Read the model definition and answer for the solid it produces. Units are mm, in the model's axes. Face numbers are marked on the shaded views. A direction names the side the tool comes from. Coordinates: 2 decimals unless noted, no trailing zeros. Write each loop counter-clockwise with the first axis right and the second up, starting at its lowest first coordinate (ties: lowest second). Pieces come first, ordered by that corner, then holes. Notation, with made-up numbers: (19, 81) -> (72, 81) arc R16 cw to (72, 101) -> close; hole circle Ø6 at (50.5, 28.5). An arc over 180 degrees is marked (long way). Use CSV: the item, a comma, the result in double quotes.
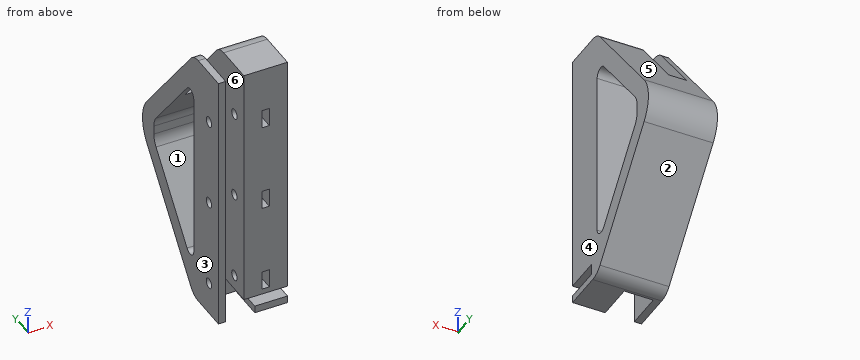
Autodesk Inventor part; units mm, degrees
ref_plane "YZ Plane" through (0, 0, 0) normal (1, 0, 0) x (0, 1, 0)
ref_plane "XZ Plane" through (0, 0, 0) normal (0, 1, 0) x (-1, 0, 0)
ref_plane "XY Plane" through (0, 0, 0) normal (0, 0, 1) x (1, 0, 0)
sketch "Sketch1" plane through (0, 0, 0) normal (0, 1, 0) x (-1, 0, 0)
  line L0 (0, 0) -> (-19, 0)
  line L1 (-19, 0) -> (-19, -73)
  line L2 (-19, -73) -> (0, -73)
  line L3 (0, -73) -> (0, 0)
  dimension "d0" = 19
  dimension "d1" = 73
extrude "Extrusion1" add sketch "Sketch1" along normal blind 13
sketch "Sketch2" plane through (19, 0, 0) normal (1, 0, 0) x (0, 0, -1)
  line L0 (0, 13) -> (0, 43) construction
  line L1 (0, 43) -> (205, 43) construction
  line L2 (0, 13) -> (0, 13.5) construction
  line L3 (0, 0) -> (0, 13) construction
  line L4 (0, 13) -> (0, 13) construction
  line L5 (0, 13) -> (73, 13) construction
  line L6 (0, 13) -> (0, 13) construction
  line L7 (0, 13) -> (73, 13) construction
  line L8 (0, 13) -> (73, 13) construction
  line L9 (36.5, 13) -> (36.5, 43) construction
  line L10 (36.5, 43) -> (0, 13) construction
  line L11 (73, 13) -> (36.5, 43) construction
  line L12 (36.5, 43) -> (30.3197, 37.9203) construction
  line L13 (30.3197, 37.9203) -> (33.4945, 34.0576) construction
  line L14 (33.4945, 34.0576) -> (7.8744, 13) construction
  line L15 (36.5, 43) -> (42.6803, 37.9203) construction
  line L16 (42.6803, 37.9203) -> (39.5055, 34.0576) construction
  line L17 (33.4945, 34.0576) -> (39.5055, 34.0576)
  line L18 (36.5, 43) -> (0, 13)
  line L19 (0, 13) -> (7.8744, 13)
  line L20 (7.8744, 13) -> (33.4945, 34.0576)
  line L21 (73, 13) -> (0, 13) construction
  line L22 (73, 13) -> (0, 13) construction
  line L23 (73, 13) -> (0, 13) construction
  line L24 (36.5, 43) -> (73, 13) construction
  line L25 (39.5055, 34.0576) -> (65.1256, 13) construction
  line L26 (36.5, 43) -> (73, 13)
  line L27 (73, 13) -> (65.1256, 13)
  line L28 (65.1256, 13) -> (39.5055, 34.0576)
  dimension "d4" = 30
  dimension "d5" = 205
  dimension "d6" = 0.5
  dimension "d7" = 0
  dimension "d8" = 0
  dimension "d9" = 73
  dimension "d10" = 0
  dimension "d11" = 8
  dimension "d12" = 5
  dimension "d13" = 8
  dimension "d14" = 5
extrude "Extrusion2" add sketch "Sketch2" against normal up to surface (19 mm away)
fillet "Fillet1" radius 10 1 edges at (9.5, 43, -36.5)
fillet "Fillet4" radius 2 2 edges at (9.5, 13, -7.8744) (9.5, 13, -65.1256)
fillet "Fillet5" radius 5 2 edges at (9.5, 13, -73) (9.5, 13, 0)
sketch "Sketch3" plane through (0, 0, 0) normal (0, -1, 0) x (1, 0, 0)
  line L0 (0, -73) -> (0, 0) construction
  line L1 (0, -73) -> (2, -73) construction
  line L2 (19, -73) -> (0, -73) construction
  line L3 (2, -73) -> (2, 0)
  line L4 (0, 0) -> (19, 0)
  line L5 (2, -73) -> (7, -73) construction
  line L6 (7, -73) -> (7, 0)
  line L7 (7, -73) -> (80, -73) construction
  line L8 (7, -73) -> (2, -73)
  line L9 (7, 0) -> (2, 0)
  dimension "d24" = 2
  dimension "d25" = 5
  dimension "d26" = 90
extrude "Extrusion3" cut sketch "Sketch3" against normal blind 10
sketch "Sketch5" plane through (0, 10, 0) normal (0, -1, 0) x (1, 0, 0)
  line L0 (7, 0) -> (7, -73)
  line L1 (2, -73) -> (2, 0)
  line L2 (7, 0) -> (2, 0)
  line L3 (2, 0) -> (2, -18)
  line L4 (2, -18) -> (7, -18)
  line L5 (7, -18) -> (7, 0)
  point P0 (0, 0)
  dimension "d31" = 18
extrude "Extrusion5" cut sketch "Sketch5" against normal up to next
sketch "Sketch6" plane through (0, 0, -73) normal (-1, 0, 0) x (0, 0, 1)
  circle A0 centre (9.0852, 5) radius 1.4
  circle A1 centre (33.5852, 5) radius 1.4
  circle A2 centre (58.0852, 5) radius 1.4
  point P0 (73, 0)
extrude "Extrusion6" cut sketch "Sketch6" against normal blind 11.995
sketch "Sketch9" plane through (11.995, 5, -14.9148) normal (-1, 0, 0) x (0, 0, 1)
  circle A0 centre (0, 0) radius 3.002 construction
  circle A1 centre (0, 0) radius 1.4 construction
  line L0 (0, 0) -> (0, 3.002) construction
  line L1 (0, 3.002) -> (2.5998, 1.501)
  line L2 (2.5998, 1.501) -> (2.5998, -1.501)
  line L3 (2.5998, -1.501) -> (0, -3.002)
  line L4 (0, -3.002) -> (-2.5998, -1.501)
  line L5 (-2.5998, -1.501) -> (-2.5998, 1.501)
  line L6 (-2.5998, 1.501) -> (0, 3.002)
  line L7 (-58.0852, -5) -> (14.9148, -5)
  line L8 (-2.5998, -1.501) -> (-2.5998, -5)
  line L9 (14.9148, -5) -> (-58.0852, -5)
  line L10 (2.5998, -1.501) -> (2.5998, -5)
  line L11 (2.5998, -1.501) -> (6.0988, -1.501) construction
  line L12 (2.5998, -5) -> (-2.5998, -5)
  dimension "d38" = 6.004
  dimension "d41" = 90
extrude "Extrusion7" cut sketch "Sketch9" against normal blind 2.005
sketch "Sketch10" plane through (14, 5, -14.9148) normal (-1, 0, 0) x (0, 0, 1)
  circle A0 centre (0, 0) radius 1.4
  line L0 (2.5998, -5) -> (-2.5998, -5)
  line L1 (2.5998, 1.501) -> (2.5998, -5)
  line L2 (0, 3.002) -> (2.5998, 1.501)
  line L3 (-2.5998, 1.501) -> (0, 3.002)
  line L4 (-2.5998, -5) -> (-2.5998, 1.501)
  point P0 (14.9148, -5)
extrude "Extrusion8" cut sketch "Sketch10" against normal blind 2 contours A0
ref_plane "Work Plane3" through (0, 5, -14.9148) normal (0, 0, -1) x (1, 0, 0)
ref_plane "Work Plane4" through (0, 5, -39.4148) normal (0, 0, 1) x (1, 0, 0)
ref_plane "Work Plane5" through (0, 5, -63.9148) normal (0, 0, -1) x (1, 0, 0)
ref_plane "Work Plane6" through (0, 5, -27.1648) normal (0, 0, -1) x (1, 0, 0)
ref_plane "Work Plane7" through (0, 5, -51.6648) normal (0, 0, 1) x (1, 0, 0)
mirror "Mirror3" about plane through (0, 5, -27.1648) normal (0, 0, -1) of "Extrusion8", "Extrusion7"
mirror "Mirror4" about plane through (0, 5, -51.6648) normal (0, 0, 1) of "Mirror3"
fillet "Fillet6" radius 5 2 edges at (9.5, 34.0576, -39.5055) (9.5, 34.0576, -33.4945)
sketch "Sketch11" plane through (0, 0, 0) normal (0, -1, 0) x (1, 0, 0)
  line L0 (7, -73) -> (2, -73) construction
  line L1 (7, -73) -> (7, -71) construction
  line L2 (7, -73) -> (9, -73) construction
  line L3 (19, -42.8497) -> (19, -71.1748)
  line L4 (7, -71) -> (19, -71)
  line L5 (19, -71) -> (19, -68)
  line L6 (19, -68) -> (7, -68)
  line L7 (7, -68) -> (7, -71)
  point P0 (0, 0)
  dimension "d48" = 2
  dimension "d49" = 90
  dimension "d50" = 3
extrude "Extrusion9" cut sketch "Sketch11" against normal blind 10
sketch "Sketch12" plane through (19, 10.6374, -73) normal (0, 0, -1) x (-1, 0, 0)
  line L0 (12, -10.6374) -> (0, -10.6374)
  line L1 (0, -0.6374) -> (12, -0.6374)
  line L2 (12, -10.6374) -> (9, -10.6374)
  line L3 (9, -10.6374) -> (9, -0.6374)
  line L4 (9, -0.6374) -> (12, -0.6374)
  line L5 (12, -0.6374) -> (12, -10.6374)
  point P0 (19, -10.6374)
  dimension "d53" = 3
extrude "Extrusion10" cut sketch "Sketch12" against normal up to next
properties part number "bumper_backright"
1. For a pull along X with two mould halves and no side action, classify the marked faces 3, 4, 5 and 6 as pulls with the +X half, pulls with the -X half, needs draft (parallel to the pull), parting line crosses it, or undercut.
Solutions:
face 3,"pulls with the -X half"
face 4,"pulls with the +X half"
face 5,"needs draft"
face 6,"undercut"
2. A cutting plane is placed at C-C (x = 8). Give the vertices of the cut face in (y, z), and give its area (3 significant figures).
Solutions:
outline,"(0, -68) -> (10, -68) -> (10, -73) -> (10.64, -73) arc R5 ccw to (14.5, -71.17) -> (37.78, -42.85) arc R10 ccw to (37.78, -30.15) -> (14.5, -1.83) arc R5 ccw to (10.64, 0) -> (0, 0) -> close; hole circle Ø2.8 at (5, -63.91); hole circle Ø2.8 at (5, -39.41); hole circle Ø2.8 at (5, -14.91); hole (13, -59.54) arc R2 ccw to (16.55, -60.81) -> (32.92, -40.89) arc R5 ccw to (34.06, -37.71) -> (34.06, -35.29) arc R5 ccw to (32.92, -32.11) -> (16.55, -12.19) arc R2 ccw to (13, -13.46) -> close"
area,"1,310 mm^2"
3. A cutting plane is placed at B-B (y = 29.5). Give the vertices of the cut face in (x, z) (3 decimals), and give its area (3 significant figures).
Solutions:
outline,"(0, -52.925) -> (19, -52.925) -> (19, -45.051) -> (0, -45.051) -> close; (0, -27.949) -> (19, -27.949) -> (19, -20.075) -> (0, -20.075) -> close"
area,"299 mm^2"
4. A cutting plane is placed at A-A (x = 4.25). Give the vertices of the cut face in (y, z), and give its area (3 significant figures).
Solutions:
outline,"(10, -73) -> (10.64, -73) arc R5 ccw to (14.5, -71.17) -> (37.78, -42.85) arc R10 ccw to (37.78, -30.15) -> (27.79, -18) -> (21.32, -18) -> (32.92, -32.11) arc R5 cw to (34.06, -35.29) -> (34.06, -37.71) arc R5 cw to (32.92, -40.89) -> (16.55, -60.81) arc R2 cw to (13, -59.54) -> (13, -18) -> (10, -18) -> close"
area,"496 mm^2"
5. Each of these flat-tipped pins is pushed along its axis until it touches: pin 1 Ø3 at (x, y) = (3, 31.5) entering from +Z; pin 2 Ø1 at (y, z) = (31.5, -45) entering from -X; pin 3 Ø2 at (y, z) = (5, -39.41) entering from -X; pin 4 Ø3.5 at (x, y) = (5.5, 12) entering from +Z. Where does it stop, or does it pass through?
Solutions:
pin 1,"stops at z = -20.68"
pin 2,"stops at x = 0"
pin 3,"stops at x = 16"
pin 4,"stops at z = -0.02"
6. Find the intervals of material crossed by line 1 along X through (y, z) = (3, -43); line 2 along Y through (x, z) = (8.25, -14.5); line 3 along Y through (x, z) = (1.25, -37.5), in increasing order.
Solutions:
line 1,"x = 0 to 2, 7 to 19"
line 2,"y = 0 to 3.66, 6.34 to 13, 18.45 to 24.92"
line 3,"y = 0 to 13, 34.06 to 40.01"
7. A cutting plane is placed at D-D (z = -50.5). Give the vertices of the cut face in (x, y).
Solutions:
outline,"(0, 0) -> (2, 0) -> (2, 10) -> (7, 10) -> (7, 0) -> (19, 0) -> (19, 13) -> (0, 13) -> close; (0, 25.02) -> (19, 25.02) -> (19, 31.49) -> (0, 31.49) -> close"
8. A tool of negligible diameter and unlimited length cuts with its end or side. For the marked faces 1 and 2, from which of +Z, -Z, +X, -X, +Y, -Y can it reach the whole face along a straight path? Write none if from no direction.
Solutions:
face 1,"+X, -X"
face 2,"-Z, +X, -X, +Y"
